```python
from build123d import *

# Parameters (mm, degrees)
ESQUISSE1_R        = 1.5
BOSS_EXTRU_1_DEPTH = 3


with BuildPart() as part:
    # Esquisse1 → Boss.-Extru.1 (new body)
    with BuildSketch(Plane.XY):
        with BuildLine():
            Line((-10.438754388, 20.283961606), (-10.438754388, -0.112631187))
            Line((-10.438754388, -0.112631187), (-10.438754388, -15.771766484))
            ThreePointArc((-10.438754388, -15.771766484), (-6.438754388, -26.243902439), (-2.438754388, -15.771766484))
            Line((-2.438754388, -15.771766484), (-2.438754388, 20.283961606))
            ThreePointArc((-2.438754388, 20.283961606), (-0.448049603, 24.422247026), (-1.966618433, 28.756097561))
            Line((-1.966618433, 28.756097561), (-2.267139353, 29.068594286))
            Line((-2.267139353, 29.068594286), (-11.126247763, 38.28073952))
            ThreePointArc((-11.126247763, 38.28073952), (-14.416088568, 40.079239654), (-18.143198107, 39.671428739))
            Line((-18.143198107, 39.671428739), (-16.826364742, 36.727346795))
            ThreePointArc((-16.826364742, 36.727346795), (-13.967550368, 36.474962725), (-12.606142543, 33.948485716))
            ThreePointArc((-12.606142543, 33.948485716), (-15.786873062, 30.92749697), (-18.640108166, 34.259533746))
            Line((-18.640108166, 34.259533746), (-21.848013666, 34.591146934))
            ThreePointArc((-21.848013666, 34.591146934), (-21.500157994, 31.799728487), (-19.963396347, 29.443590936))
            Line((-19.963396347, 29.443590936), (-10.751251112, 20.584482526))
            Line((-10.751251112, 20.584482526), (-10.438754388, 20.283961606))
        make_face()
        with Locations((-6.438754388, -20.243902439)):
            Circle(ESQUISSE1_R, mode=Mode.SUBTRACT)
        with Locations((-6.438754388, 24.756097561)):
            Circle(ESQUISSE1_R, mode=Mode.SUBTRACT)
    extrude(amount=BOSS_EXTRU_1_DEPTH)


solid = part.part
```
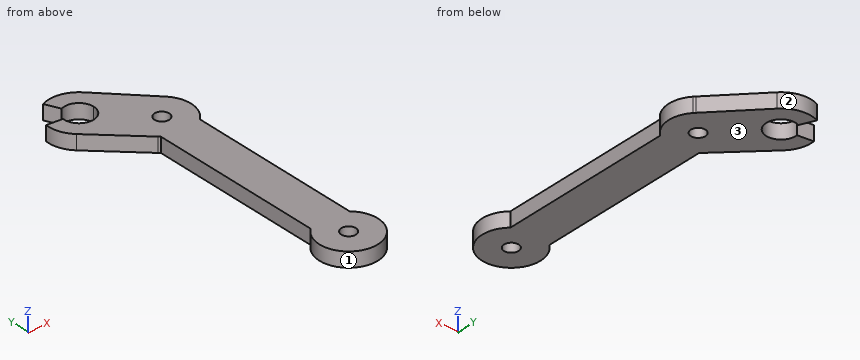
Work out the finished part from the listing and answer in its coordinate system (mm). Face numbers are marked on the shaded views. Give positions to 0.01 mm unless a question says otherwise; leave off trailing zeros. Loops run counter-clockwise (first coordinate to the right, second up) from the corner with the lowest first, then second, coordinate; pieces in that order, holes last. Notation, with made-up numbers: (81, 11.5) -> (121, 11.5) arc R38 cw to (121, 49.5) -> close; hole circle Ø6 at (63.5, 78.5). An arc over 180 degrees is marked (long way). Put each result on its own line as item: value. Start each with the question number.
Item 1: The part is cut by section C-C (x = -6.75). Give the vertices of the cut face in (y, z).
Item 2: The part is cut by section D-D (y = 0). Give the vertices of the cut face in (x, z), then the cut area to 3 significant figures.
Item 3: The part is cut by section A-A (x = -14). Give the vertices of the cut face in (y, z), then the cut area to 3 significant figures.
Item 4: The mould has two halves that part along Y. Classify the marked faces 1, 2 and 3: released by +Y, released by -Y, zero draft, split by the parting line, or undercut.
Item 5: The part is cut by section B-B (z = 0.55). Give the vertices of the cut face in (x, y) (3 decimals), then the cut area to 3 significant figures.
Item 6: Find the intervals of material crossed by L1, parallel to Y at x = -6, z = 1.15; L2, parallel to Y at x = -6.5, z = 0.2; L3, parallel to X at y = -4.5, z = 2.1, in increasing order. Write a range as [from, to].
Item 7: This flat-tipped pin is pushed along its axis until it touches: P1, Ø0.9, axis at y = 0.5, z = 1.5, coming from the -X side. Where does it stop, or does it pass through?
Answers below:
1. outline: (-26.24, 0) -> (-21.71, 0) -> (-21.71, 3) -> (-26.24, 3) -> close; (-18.78, 0) -> (23.29, 0) -> (23.29, 3) -> (-18.78, 3) -> close; (26.22, 0) -> (33.73, 0) -> (33.73, 3) -> (26.22, 3) -> close
2. outline: (-10.44, 0) -> (-2.44, 0) -> (-2.44, 3) -> (-10.44, 3) -> close
2. area: 24.0 mm2
3. outline: (23.71, 0) -> (31.4, 0) -> (31.4, 3) -> (23.71, 3) -> close; (36.5, 0) -> (39.98, 0) -> (39.98, 3) -> (36.5, 3) -> close
3. area: 33.5 mm2
4. face 1: undercut
4. face 2: released by +Y
4. face 3: zero draft
5. outline: (-21.848, 34.591) arc R6.25 ccw to (-19.963, 29.444) -> (-10.439, 20.284) -> (-10.439, -15.772) arc R6 ccw (long way) to (-2.439, -15.772) -> (-2.439, 20.284) arc R6 ccw to (-1.967, 28.756) -> (-11.126, 38.281) arc R6.25 ccw to (-18.143, 39.671) -> (-16.826, 36.727) arc R3.025 cw (long way) to (-18.64, 34.26) -> close; hole circle Ø3 at (-6.439, -20.244); hole circle Ø3 at (-6.439, 24.756)
5. area: 603 mm2
6. L1: [-26.23, -21.68], [-18.81, 23.32], [26.19, 32.95]
6. L2: [-26.24, -21.74], [-18.75, 23.26], [26.25, 33.47]
6. L3: [-10.44, -2.44]
7. P1: x = -10.44
